Autodesk Inventor part; units mm, degrees
ref_plane "YZ Plane" through (0, 0, 0) normal (1, 0, 0) x (0, 1, 0)
ref_plane "XZ Plane" through (0, 0, 0) normal (0, 1, 0) x (-1, 0, 0)
ref_plane "XY Plane" through (0, 0, 0) normal (0, 0, 1) x (1, 0, 0)
sketch "Sketch1" plane through (0, 0, 0) normal (0, 0, 1) x (1, 0, 0)
  circle A0 centre (0, 0) radius 3
  dimension "d0" = 6
extrude "Extrusion1" add sketch "Sketch1" along normal blind 1.5
sketch "Sketch2" plane through (0, 0, 1.5) normal (0, 0, 1) x (1, 0, 0)
  circle A0 centre (0, 0) radius 3 construction
  circle A1 centre (0, 0) radius 1.5
  dimension "d3" = 3
extrude "Extrusion2" add sketch "Sketch2" along normal blind 3
sketch "Sketch3" plane through (0, 0, 0) normal (0, 0, -1) x (-1, 0, 0)
  circle A0 centre (0, 0) radius 1.5
  dimension "d6" = 3
extrude "Extrusion3" add sketch "Sketch3" along normal blind 3
thread "Thread1"
thread "Thread2"
chamfer "Chamfer1" distance 0.1 angle 45 1 edges at (-3, 0, 1.5)
chamfer "Chamfer2" distance 0.1 angle 45 1 edges at (-3, 0, 0)
properties part number "threaded_coupler_m3x05_r01"
Could you check a few things on this model? Use its own coordinates, in mm. A direction names the side the tool comes from. Give positions to 0.01 mm unless a question says otherwise; leave off trailing zeros. Loops run counter-clockwise (first coordinate to the right, second up) from the corner with the lowest first, then second, coordinate; pieces in that order, holes last. Notation, with made-up numbers: (-25, -2) - (17, -2) arc R27 ccw to (17, 17) - close; hole circle Ø9 at (-35.75, 33.5). An arc over 180 degrees is marked (long way). Answer in a Markdown table with one row per item. Add a question column.
Q1. Please list where these lines run through material, in increasing order: L1, parallel to Z at x = 0.95, y = 1.7; L2, parallel to X at y = -0.85, z = -1; L3, parallel to Y at x = 0.8, z = 2. Write a range as from..to.
Q2. If we section it at A-A (y = 0): List the corners of the cut face in (x, z) for me.
Q3. If we section it at C-C (z = 0.5): List the corners of the cut face in (x, y) for me, plus the area to 3 significant figures.
Q4. Which directions (+Z, -Z, +X, -X, +Y, -Y) give clear straight access to the entire face, cutting with the end or side of a thin tool? Please do faces 1 (the face through (1.2, -1.2, 1.5)), 2 (the face through (1.2, -1.2, 0)), 3 (the face through (0, 0, -3)).
Q5. If we section it at D-D (z = 3): List the corners of the cut face in (x, y) for me, plus the area to 3 significant figures.
Q6. For pin 1 (1.5 mm diameter, centred on y = -2, z = -2, fed in from -X); pin 2 (2 mm diameter, centred on x = 2, z = 1.5, fed in from +Y); pin 3 (1.5 mm diameter, centred on x = -0.5, z = 2.5, fed in from +Y), each with a flat end and sliding along its axis, tell me the tip position at first contact or that it passes through.
The answers:
| question | item | result |
|---|---|---|
| 1 | L1 | z = 0..1.5 |
| 1 | L2 | x = -1.24..1.24 |
| 1 | L3 | y = -1.27..1.27 |
| 2 | outline | (-3, 0.1) - (-2.9, 0) - (-1.5, 0) - (-1.5, -3) - (1.5, -3) - (1.5, 0) - (2.9, 0) - (3, 0.1) - (3, 1.4) - (2.9, 1.5) - (1.5, 1.5) - (1.5, 4.5) - (-1.5, 4.5) - (-1.5, 1.5) - (-2.9, 1.5) - (-3, 1.4) - close |
| 3 | outline | circle Ø6 at (0, 0) |
| 3 | area | 28.3 mm^2 |
| 4 | face 1 | +Z |
| 4 | face 2 | -Z |
| 4 | face 3 | -Z, +X, -X, +Y, -Y |
| 5 | outline | circle Ø3 at (0, 0) |
| 5 | area | 7.07 mm^2 |
| 6 | pin 1 | stops at x = -0.83 |
| 6 | pin 2 | stops at y = 2.83 |
| 6 | pin 3 | stops at y = 1.5 |
